The listing builds one solid part. Answer for the finished solid, in the listing's coordinates (mm). Round coordinates to 2 decimals unless told otherwise and drop trailing zeros. Write each loop counter-clockwise with the first axis right and the second up, starting at its lowest first coordinate (ties: lowest second). Pieces come first, ordered by that corner, then holes. Notation, with made-up numbers: M -29,64 L -18,64 A35 ccw -18,101 Z; hole C -35.5,-7.5 d3. An arc over 180 degrees is marked long. Put each result on its own line as item: value. Start each with the question number.
Autodesk Inventor part; units mm, degrees
ref_plane "YZ Plane" through (0, 0, 0) normal (1, 0, 0) x (0, 1, 0)
ref_plane "XZ Plane" through (0, 0, 0) normal (0, 1, 0) x (-1, 0, 0)
ref_plane "XY Plane" through (0, 0, 0) normal (0, 0, 1) x (1, 0, 0)
sketch "Sketch1" plane through (0, 0, 0) normal (0, 1, 0) x (-1, 0, 0)
  circle A0 centre (50.4794, -84.4325) radius 1.6
  circle A1 centre (-50.4794, -84.4325) radius 1.6
  arc A2 (50.4794, -89.4325) -> (50.4794, -79.4325) centre (50.4794, -84.4325) ccw
  arc A3 (-50.4794, -79.4325) -> (-50.4794, -89.4325) centre (-50.4794, -84.4325) ccw
  line L0 (50.4794, -79.4325) -> (-50.4794, -79.4325)
  line L1 (-50.4794, -89.4325) -> (50.4794, -89.4325)
  point P0 (0, 0)
  dimension "d0" = 3.2
  dimension "d1" = 3.2
  dimension "d2" = 5
  dimension "d3" = 5
extrude "Extrusion1" add sketch "Sketch1" along normal blind 3
properties part number "Front guard"
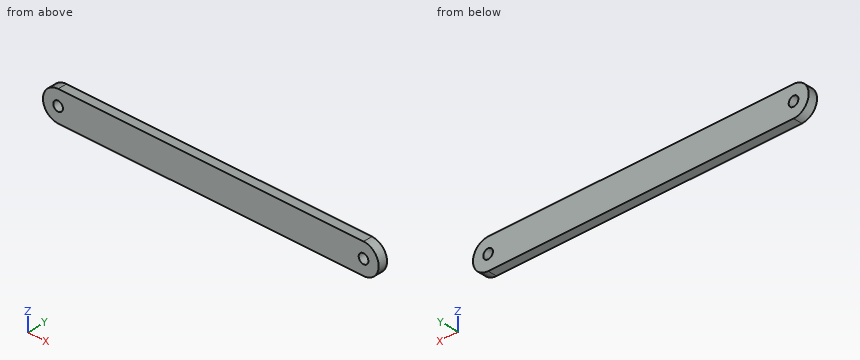
Item 1: Section B-B (z = -80.5) is taken. Give the vertices of the cut face in (x, y).
Item 2: Section A-A (y = 2.3) is taken. Give the vertices of the cut face in (x, z).
Item 3: Consider line 1 along X through (y, z) = (0.9, -84); line 2 along Z through (x, y) = (-50.5, 1.8); line 3 along X through (y, z) = (0.6, -85.5). Determine where each line is inside the solid, lowest interval first. Write a range as [from, to].
Output values:
1. outline: M -53.57,0 L 53.57,0 L 53.57,3 L -53.57,3 Z
2. outline: M -50.48,-89.43 L 50.48,-89.43 A5 ccw 50.48,-79.43 L -50.48,-79.43 A5 ccw Z; hole C -50.48,-84.43 d3.2; hole C 50.48,-84.43 d3.2
3. line 1: x = [-55.46, -52.02], [-48.94, 48.94], [52.02, 55.46]
3. line 2: z = [-89.43, -86.03], [-82.83, -79.43]
3. line 3: x = [-55.36, -51.67], [-49.29, 49.29], [51.67, 55.36]
